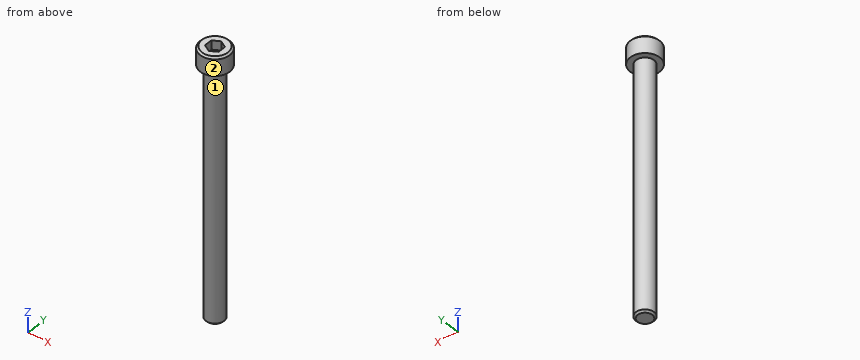
Autodesk Inventor part; units mm, degrees
ref_plane "YZ Plane" through (0, 0, 0) normal (1, 0, 0) x (0, 1, 0)
ref_plane "XZ Plane" through (0, 0, 0) normal (0, 1, 0) x (-1, 0, 0)
ref_plane "XY Plane" through (0, 0, 0) normal (0, 0, 1) x (1, 0, 0)
sketch "Sketch1" plane through (0, 0, 0) normal (0, 0, 1) x (1, 0, 0)
  circle A0 centre (0, 0) radius 4
  dimension "Diameter" = 8
extrude "Extrusion1" add sketch "Sketch1" along normal blind 110
sketch "Sketch2" plane through (0, 0, 110) normal (0, 0, 1) x (1, 0, 0)
  circle A0 centre (0, 0) radius 4
  circle A1 centre (0, 0) radius 6.5
  dimension "Head_Diameter" = 13
extrude "Extrusion2" add sketch "Sketch2" along normal blind 8 contours A0 | A1
sketch "Sketch3" plane through (0, 0, 118) normal (0, 0, 1) x (1, 0, 0)
  circle A0 centre (0, 0) radius 6.5
  circle A1 centre (0, 0) radius 3.4641 construction
  line L0 (0, 3.4641) -> (3, 1.7321)
  line L1 (3, -1.7321) -> (3, 1.7321)
  line L2 (0, 3.4641) -> (-3, 1.7321)
  line L3 (-3, -1.7321) -> (-3, 1.7321)
  line L4 (-3, -1.7321) -> (0, -3.4641)
  line L5 (3, -1.7321) -> (0, -3.4641)
  dimension "Hex_Width" = 6
extrude "Extrusion3" cut sketch "Sketch3" against normal blind 4 contours L0 L1 L5 L4 L3 L2
thread "Thread1"
chamfer "Chamfer1" distance 0.8 angle 45 2 edges at (-6.5, 0, 118) (-4, 0, 0)
equation "\"d9\" = ThreadLength"
equation "\"d12\" = Chamfer"
equation "\"ThreadLength\" = 28"
properties part number "SCREW, SOCKET HD, P, 12.9, M8X1.25X110MM"
The model under review builds one solid part; all positions refer to its coordinate system, in mm. Face numbers are marked on the shaded views. A direction names the side the tool comes from. Round coordinates to 2 decimals unless told otherwise and drop trailing zeros. Loops run counter-clockwise (first coordinate to the right, second up) from the corner with the lowest first, then second, coordinate; pieces in that order, holes last. Notation, with made-up numbers: M 79.5,84.5 L 95.5,84.5 A25 ccw 95.5,113.5 Z; hole C 18,8 d4. An arc over 180 degrees is marked long. Put each result on its own line as item: value.
Q1. Consider section A-A, the plane y = 0. Give the boundary of the cut face in (x, z), then the cut area to 3 significant figures.
Result set:
outline: M -6.5,110 L -4,110 L -4,0.8 L -3.2,0 L 3.2,0 L 4,0.8 L 4,110 L 6.5,110 L 6.5,117.2 L 5.7,118 L 3,118 L 3,114 L -3,114 L -3,118 L -5.7,118 L -6.5,117.2 Z
area: 959 mm²
Q2. To check wall thickness, follow L1, parallel to Z at x = 0.75, y = -3; L2, parallel to Z at x = -4.5, y = -3; L3, parallel to X at y = 2, z = 91. State the ranges of each line that lie inside material, in increasing order.
Result set:
L1: z = 0 to 114
L2: z = 110 to 118
L3: x = -3.46 to 3.46
Q3. Consider section B-B, the plane z = 79. Give the boundary of the cut face in (x, y), then the cut area to 3 significant figures.
Result set:
outline: C 0,0 d8
area: 50.3 mm²
Q4. Machinability: for the marked faces 1 and 2, which of the approach directions +Z, -Z, +X, -X, +Y, -Y give a long, thin tool a straight path to every point of the face, cutting with its end or side? Answer none if there is none.
Result set:
face 1: -Z
face 2: +Z, -Z
Q5. For pin 1 (1 mm diameter, centred on y = -5, z = 75, fed in from +X); pin 2 (2 mm diameter, centred on y = 3.5, z = 74.5, fed in from +X); pin 3 (6 mm diameter, centred on x = 0.5, z = 74, fed in from -Y), all flat-tipped, find the tip position at first contact; note any pin that passes through.
Result set:
pin 1: passes through
pin 2: stops at x = 3.12
pin 3: stops at y = -4
